Autodesk Inventor part; units mm, degrees
ref_plane "Work Plane1" through (0, 0, 0) normal (-0.7071, 0.7071, 0) x (0, 0, 1)
ref_plane "YZ Plane" through (0, 0, 0) normal (1, 0, 0) x (0, 1, 0)
ref_plane "XY Plane" through (0, 0, 0) normal (0, 0, 1) x (1, 0, 0)
sketch "Sketch1" plane through (0, 0, 0) normal (0, 0, 1) x (1, 0, 0)
  circle A0 centre (0, 0) radius 8.5
  dimension "d0" = 17
extrude "Extrusion1" add sketch "Sketch1" along normal blind 8
sketch "Sketch2" plane through (0, 0, 8) normal (0, 0, 1) x (1, 0, 0)
  circle A0 centre (0, 0) radius 7.7
  circle A1 centre (0, 0) radius 8.5
  dimension "d3" = 0.8
extrude "Extrusion2" cut sketch "Sketch2" against normal blind 6.8 contours A0
sketch "Sketch3" plane through (0, 0, 0) normal (0, 0, -1) x (-1, 0, 0)
  point P0 (0, 0)
hole "Hole1" at (0, 0, 0) direction (0, 0, 1) diameter 3.2 end through all
sketch "Sketch4" plane through (0, 0, 1.2) normal (0, 0, 1) x (1, 0, 0)
  circle A0 centre (0, 0) radius 1.6
  circle A1 centre (0, 0) radius 7.7
  line L0 (-11.9, 0) -> (11.9, 0)
  line L1 (0, -11.9) -> (0, 11.9)
  circle A2 centre (0, 0) radius 3.6
  circle A3 centre (0, 0) radius 4.9
  line L2 (0, 0) -> (2.45, 4.2435)
  line L3 (0, 0) -> (4.2435, 2.45)
  point P0 (0, 7.7)
  point P1 (0, 1.6)
  point P2 (1.6, 0)
  point P3 (7.7, 0)
  point P4 (3.6, 0)
  point P5 (3.1177, 1.8)
  point P6 (4.9, 0)
  point P7 (0, 4.9)
  point P8 (1.8, 3.1177)
  point P9 (0, 3.6)
  dimension "d15" = 30
  dimension "d16" = 30
  dimension "d17" = 9.8
  dimension "d18" = 7.2
extrude "Extrusion3" add sketch "Sketch4" along normal blind 2 contours A0 L3 A2 L0 | A0 L2 A2 L3 | A0 L1 A2 L2 | A2 L2 A3 L3 | A3 L1 A1 L0 picked at (4.6569, 4.8582)
extrude "Extrusion4" add sketch "Sketch4" along normal blind 3 contours L0 A2 L1 A0 | A0 L3 A2 L0 | A0 L2 A2 L3 | L1 A2 L0 A0 | A0 L1 A2 L2 | L0 A2 L1 A0
sketch "Sketch5" plane through (1.8, 3.1177, 1.2) normal (-0.866, 0.5, 0) x (0, 0, 1)
  line L0 (0, 0) -> (0, 1.3)
  line L1 (0, 0) -> (2, 0)
  line L2 (2, 1.3) -> (2, 0)
  line L3 (0, 1.3) -> (2, 1.3)
  circle A0 centre (0.65, 0.65) radius 0.65
  line L4 (0, 1.3) -> (2, 1.3)
  line L5 (0, 0) -> (2, 0)
  line L6 (-2.8, -3.6) -> (8.4, -3.6)
  point P0 (-1.2, -3.6)
revolve "Revolution1" cut sketch "Sketch5" angle 10 about axis through (0, 0, -10) along (0, 0, -1) contours A0
ref_plane "Work Plane1" through (0, 0, 0) normal (-0.7071, 0.7071, 0) x (0, 0, 1)
mirror "Mirror1" about plane through (0, 0, 0) normal (-0.7071, 0.7071, 0) of "Revolution1"
properties part number "RewingingSpoolBushing"
Geometry check sheet. Reference: the model listing, model coordinates, mm. A direction names the side the tool comes from. Round coordinates to 2 decimals unless told otherwise and drop trailing zeros. Order: outer loops, then holes, each group sorted by start corner. A loop starts at its lowest first (then second) coordinate and runs counter-clockwise, first axis right, second up. Notation, with made-up numbers: M 58,44.25 L 109,44.25 A15 ccw 109,56.25 Z; hole C -32,34.25 d4. An arc over 180 degrees is marked long. Write each question's results on one line, items separated by ' | '. Start each with the question number.
1. Draft check along X on faces 1 (the face through (-1, 8, 8)), 2 (the face through (4.57, -7.167, 3.944)), 3 (the face through (2, -1, 4.2)). Enter one of: pulls with the +X half, pulls with the -X half, needs draft (parallel to the pull), parting line crosses it, or undercut.
2. Set-up check for faces 4 (the face through (2, 0, 0)), 5 (the face through (4.728, 1.286, 2.186)), 6 (the face through (2.738, 3.263, 1.841)): record each of +Z, -Z, +X, -X, +Y, -Y from which the full face is reachable in a straight line by a thin tool's end or side.
3. Cross-section at B-B on z = 3.5. Record the boundary of the cut face in (x, y), plus the area to 3 significant figures.
4. Cross-section at D-D on z = 7.75. Record the boundary of the cut face in (x, y), plus the area to 3 significant figures.
5. Cross-section at A-A on y = -0.5. Record the boundary of the cut face in (x, z), plus the area to 3 significant figures.
6. Go/stop test with flat-tipped pins: P1, Ø1.5, axis at y = -6.5, z = 1.5, coming from the +X side; P2, Ø1, axis at x = 2.5, y = -4, coming from the +Z side; P3, Ø4.5, axis at x = -0.5, y = -0.5, coming from the +Z side; P4, Ø1.9, axis at x = 0, y = 0, coming from the +Z side. Record where each tip stops, or that it passes through.
7. Material ranges on L1, parallel to Y at x = 0, z = 0.4; L2, parallel to Y at x = -0.75, z = 4; L3, parallel to Y at x = 0, z = 6, recorded low to high. Write a range as from..to.
8. Cross-section at C-C on x = -7.25. Record the boundary of the cut face in (y, z), plus the area to 3 significant figures.
Resolved:
1) face 1: needs draft | face 2: parting line crosses it | face 3: undercut
2) face 4: -Z, +X, -X, +Y, -Y | face 5: +Z | face 6: none
3) outline: C 0,0 d17; C 0,0 d7.2; hole C 0,0 d15.4; hole C 0,0 d3.2 | area: 73.4 mm2
4) outline: C 0,0 d17; hole C 0,0 d15.4 | area: 40.7 mm2
5) outline: M -8.49,0 L -1.52,0 L -1.52,4.2 L -3.57,4.2 L -3.57,1.2 L -7.68,1.2 L -7.68,8 L -8.49,8 Z; M 1.52,0 L 8.49,0 L 8.49,8 L 7.68,8 L 7.68,1.2 L 3.57,1.2 L 3.57,4.2 L 1.52,4.2 Z | area: 39.9 mm2
6) P1: x = 6.26 | P2: z = 1.2 | P3: z = 4.2 | P4: through
7) L1: -8.5..-1.6, 1.6..8.5 | L2: -8.47..-7.66, -3.52..-1.41, 1.41..3.52, 7.66..8.47 | L3: -8.5..-7.7, 7.7..8.5
8) outline: M -4.44,0 L 4.44,0 L 4.44,8 L 2.59,8 L 2.59,1.2 L -2.59,1.2 L -2.59,8 L -4.44,8 Z | area: 35.7 mm2
